The model under review builds one solid part; all positions refer to its coordinate system, in mm. Round coordinates to 2 decimals unless told otherwise and drop trailing zeros. Loops run counter-clockwise (first coordinate to the right, second up) from the corner with the lowest first, then second, coordinate; pieces in that order, holes last. Notation, with made-up numbers: M 18.25,82 L 42.25,82 A26 ccw 42.25,109 Z; hole C 85.5,73 d6. An arc over 180 degrees is marked long. Use a Markdown table: item, result. Add a question column.
```python
from build123d import *

# Parameters (mm, degrees)
CROQUIS1_W              = 200
CROQUIS1_H              = 200
CROQUIS1_R              = 2.5
SALIENTE_EXTRUIR1_DEPTH = 4
CROQUIS2_W              = 158
CROQUIS2_H              = 158
CORTAR_EXTRUIR1_DEPTH   = 10
CROQUIS3_W              = 200
CROQUIS3_H              = 200
CROQUIS3_W_2            = 180
CROQUIS3_H_2            = 180
CORTAR_EXTRUIR2_DEPTH   = 10
CROQUIS4_W              = 158
CROQUIS4_H              = 5
CROQUIS4_W_2            = 5
CROQUIS4_H_2            = 158
SALIENTE_EXTRUIR2_DEPTH = 5
CROQUIS5_W              = 162
CROQUIS5_H              = 162
CROQUIS5_W_2            = 158
CROQUIS5_H_2            = 158
CORTAR_EXTRUIR4_DEPTH   = 5


with BuildPart() as part:
    # Croquis1 → Saliente-Extruir1 (new body)
    with BuildSketch(Plane(origin=(0, 0, 0), x_dir=(1, 0, 0), z_dir=(0, 1, 0))):
        with Locations((100, 100)):
            Rectangle(CROQUIS1_W, CROQUIS1_H)
        with Locations(Location((15, 185, 0), (0, 0, 270))):
            Circle(CROQUIS1_R, mode=Mode.SUBTRACT)
        with Locations(Location((185, 185, 0), (0, 0, 270))):
            Circle(CROQUIS1_R, mode=Mode.SUBTRACT)
        with Locations(Location((185, 15, 0), (0, 0, 270))):
            Circle(CROQUIS1_R, mode=Mode.SUBTRACT)
        with Locations(Location((15, 15, 0), (0, 0, 270))):
            Circle(CROQUIS1_R, mode=Mode.SUBTRACT)
    extrude(amount=SALIENTE_EXTRUIR1_DEPTH)

    # Croquis2 → Cortar-Extruir1 (cut)
    with BuildSketch(Plane(origin=(0, 4, 0), x_dir=(1, 0, 0), z_dir=(0, 1, 0))):
        with Locations((100, 100)):
            Rectangle(CROQUIS2_W, CROQUIS2_H)
    extrude(amount=-CORTAR_EXTRUIR1_DEPTH, mode=Mode.SUBTRACT)

    # Croquis3 → Cortar-Extruir2 (cut)
    with BuildSketch(Plane(origin=(0, 4, 0), x_dir=(1, 0, 0), z_dir=(0, 1, 0))):
        with Locations((100, 100)):
            Rectangle(CROQUIS3_W, CROQUIS3_H)
        with Locations((100, 100)):
            Rectangle(CROQUIS3_W_2, CROQUIS3_H_2, mode=Mode.SUBTRACT)
    extrude(amount=-CORTAR_EXTRUIR2_DEPTH, mode=Mode.SUBTRACT)

    # Croquis4 → Saliente-Extruir2 (add)
    with BuildSketch(Plane(origin=(0, 4, 0), x_dir=(1, 0, 0), z_dir=(0, 1, 0))):
        with Locations((100, 187.5)):
            Rectangle(CROQUIS4_W, CROQUIS4_H)
        with Locations((187.5, 100)):
            Rectangle(CROQUIS4_W_2, CROQUIS4_H_2)
        with Locations((100, 12.5)):
            Rectangle(CROQUIS4_W, CROQUIS4_H)
        with Locations((12.5, 100)):
            Rectangle(CROQUIS4_W_2, CROQUIS4_H_2)
    extrude(amount=SALIENTE_EXTRUIR2_DEPTH)

    # Croquis5 → Cortar-Extruir4 (cut)
    with BuildSketch(Plane(origin=(0, 4, 0), x_dir=(1, 0, 0), z_dir=(0, 1, 0))):
        with Locations((100, 100)):
            Rectangle(CROQUIS5_W, CROQUIS5_H)
        with Locations((100, 100)):
            Rectangle(CROQUIS5_W_2, CROQUIS5_H_2, mode=Mode.SUBTRACT)
    extrude(amount=-CORTAR_EXTRUIR4_DEPTH, mode=Mode.SUBTRACT)


solid = part.part
```
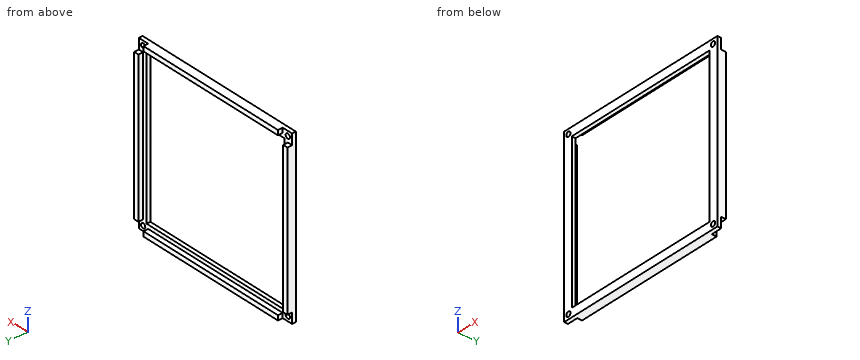
(1) Consider section B-B, the plane z = -148. Give the boundary of the cut face in (x, y).
(2) Consider section C-C, the plane x = 69. Give the boundary of the cut face in (y, z).
(3) Consider section A-A, the plane y = 6.5. Give the boundary of the cut face in (x, z), then the cut area to 3 significant figures.
(4) To check wall thickness, follow probe 1 along X at (y, z) = (2.6, -15); probe 2 along Z at (x, y) = (185, 2.3); probe 3 along Z at (x, y) = (122, 5.5). State the ranges of each line that lie inside material, in increasing order.
(5) Insertion check: pin 1 Ø6.5 at (x, z) = (15, -185) entering from +Y; pin 2 Ø4 at (y, z) = (7.5, -12.5) entering from +X; pin 3 Ø1.5 at (x, y) = (188.5, 6.5) entering from +Z. Each pin has a flat end and moves straight along its axis. Give the tip position at first contact, or say it passes through.
Found:
| question | item | result |
|---|---|---|
| 1 | outline | M 10,0 L 19,0 L 19,4 L 15,4 L 15,9 L 10,9 Z; M 181,0 L 190,0 L 190,9 L 185,9 L 185,4 L 181,4 Z |
| 2 | outline | M 0,-190 L 9,-190 L 9,-185 L 4,-185 L 4,-181 L 0,-181 Z; M 0,-19 L 4,-19 L 4,-15 L 9,-15 L 9,-10 L 0,-10 Z |
| 3 | outline | M 10,-179 L 15,-179 L 15,-21 L 10,-21 Z; M 21,-190 L 179,-190 L 179,-185 L 21,-185 Z; M 21,-15 L 179,-15 L 179,-10 L 21,-10 Z; M 185,-179 L 190,-179 L 190,-21 L 185,-21 Z |
| 3 | area | 3,160 mm^2 |
| 4 | probe 1 | x = 10 to 12.5, 17.5 to 182.5, 187.5 to 190 |
| 4 | probe 2 | z = -190 to -187.5, -182.5 to -17.5, -12.5 to -10 |
| 4 | probe 3 | z = -190 to -185, -15 to -10 |
| 5 | pin 1 | stops at y = 4 |
| 5 | pin 2 | stops at x = 179 |
| 5 | pin 3 | stops at z = -21 |
